```python
from build123d import *

# Parameters (mm, degrees)
SKETCH_1_W          = 60
SKETCH_1_H          = 90
EXTRUDE_1_DEPTH     = 21
SKETCH_2_R          = 2.5
CUT_EXTRUDE_1_DEPTH = 5
FILLET_2_R          = 2


with BuildPart() as part:
    # 草图1 → 凸台-拉伸1 (new body)
    with BuildSketch(Plane(origin=(0, 0, 0), x_dir=(0, 0, -1), z_dir=(1, 0, 0))):
        with Locations((-30, -45)):
            Rectangle(SKETCH_1_W, SKETCH_1_H)
    extrude(amount=EXTRUDE_1_DEPTH)

    # 草图2 → 切除-拉伸1 (cut)
    with BuildSketch(Plane(origin=(0, 0, 0), x_dir=(-1, 0, 0), z_dir=(0, 0, -1))):
        with Locations(Location((-10.5, -10, 0), (0, 0, 90))):
            Circle(SKETCH_2_R)
    extrude(amount=-CUT_EXTRUDE_1_DEPTH, mode=Mode.SUBTRACT)

    # 圆角2
    fillet_2_edges = [part.edges().sort_by_distance(p)[0] for p in [
        (21, -45, 60),
        (10.5, -12.5, 0),
        (21, -90, 30),
        (21, -45, 0),
        (0, -90, 30),
        (0, -45, 60),
        (0, 0, 30),
        (0, -45, 0),
        (10.5, -90, 0),
        (10.5, -90, 60),
        (10.5, 0, 60),
        (10.5, 0, 0),
        (21, 0, 30),
    ]]
    fillet(fillet_2_edges, radius=FILLET_2_R)


solid = part.part
```
CAD build for the part. Positions are in the model's coordinates, mm. A direction names the side the tool comes from. Round coordinates to 2 decimals unless told otherwise and drop trailing zeros. Order: outer loops, then holes, each group sorted by start corner. A loop starts at its lowest first (then second) coordinate and runs counter-clockwise, first axis right, second up. Notation, with made-up numbers: (0, 43.5) -> (16, 43.5) arc R16 ccw to (16, 68.5) -> close; hole circle Ø3 at (38.25, 28). An arc over 180 degrees is marked (long way). Write item = value, one per line.
(1) Drill centre lines: L1, parallel to X at y = -10, z = 4; L2, parallel to Z at x = 1.5, y = -37; L3, parallel to Y at x = 19.5, z = 42. Where is each one in solid material? Low to high.
Answers follow:
L1 = 0 to 8, 13 to 21
L2 = 0.06 to 59.94
L3 = -89.94 to -0.06
(2) 3-axis set-ups, long thin cutter, end or side, ignore diameter. For faces 4 (the flat face through (11, -10, 5)), 5 (the flat face through (10, -90, 30)): which of +Z, -Z, +X, -X, +Y, -Y reach the whole face in a straight line?
Answers follow:
face_4 = -Z
face_5 = +Z, -Z, +X, -X, -Y
(3) Pull direction X, two halves, no side cores. Call faces 1 (the cylindrical face through (8.06, -10.54, 3.48)), 2 (the flat face through (10, -46, 0)), 3 (the cylindrical face through (0.6, -44.4, 59.43)): +X half, -X half, draft (parallel to the pull), parting line (faces both ways), or undercut.
Answers follow:
face_1 = undercut
face_2 = draft
face_3 = -X half
(4) Flat gauge pins, fed straight in: P1, Ø5.5, axis at x = 10.5, y = -9.5, coming from the -Z side; P2, Ø3, axis at x = 10.5, y = -10, coming from the -Z side. Where does each tip first touch, or does it go through?
Answers follow:
P1 = 0.44
P2 = 5
(5) Cut at A-A (y = -10). Write the cut outline in (x, z).
Answers follow:
outline = (0, 2) arc R2 ccw to (2, 0) -> (6, 0) arc R2 ccw to (8, 2) -> (8, 5) -> (13, 5) -> (13, 2) arc R2 ccw to (15, 0) -> (19, 0) arc R2 ccw to (21, 2) -> (21, 58) arc R2 ccw to (19, 60) -> (2, 60) arc R2 ccw to (0, 58) -> close
